Read the model definition and answer for the solid it produces. Units are mm, in the model's axes. Face numbers are marked on the shaded views. A direction names the side the tool comes from. Coordinates: 2 decimals unless noted, no trailing zeros. Write each loop counter-clockwise with the first axis right and the second up, starting at its lowest first coordinate (ties: lowest second). Pieces come first, ordered by that corner, then holes. Notation, with made-up numbers: (8, 8) -> (44, 8) arc R6 cw to (44, 15) -> close; hole circle Ø7 at (31.25, -17.5). An arc over 180 degrees is marked (long way). Return JSON: item names as keys, results as strings.
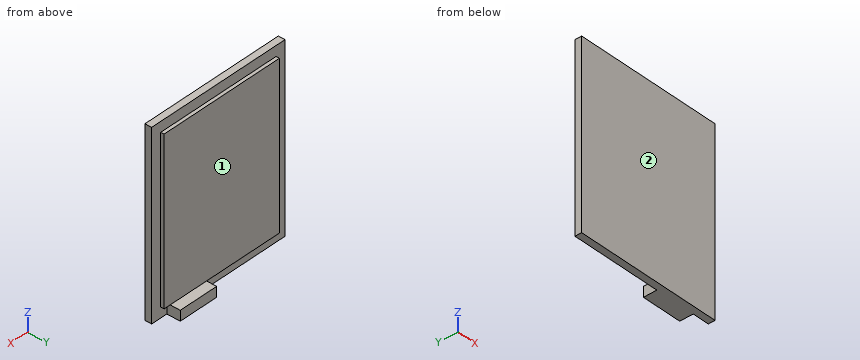
from build123d import *

# Parameters (mm, degrees)
SCHIZZO1_W                   = 44
SCHIZZO1_H                   = 54
ESTRUSIONE_ESTRUSIONE1_DEPTH = 2
SCHIZZO2_W                   = 38
SCHIZZO2_H                   = 48
ESTRUSIONE_ESTRUSIONE2_DEPTH = 1
SCHIZZO3_W                   = 12
SCHIZZO3_H                   = 3
ESTRUSIONE_ESTRUSIONE3_DEPTH = 4


with BuildPart() as part:
    # Schizzo1 → Estrusione-Estrusione1 (new body)
    with BuildSketch(Plane(origin=(0, 0, 0), x_dir=(1, 0, 0), z_dir=(0, 1, 0))):
        with Locations((9.928073705, -8.029830108)):
            Rectangle(SCHIZZO1_W, SCHIZZO1_H)
    extrude(amount=ESTRUSIONE_ESTRUSIONE1_DEPTH)

    # Schizzo2 → Estrusione-Estrusione2 (add)
    with BuildSketch(Plane(origin=(0, 2, 0), x_dir=(1, 0, 0), z_dir=(0, 1, 0))):
        with Locations((9.928073705, -8.029830108)):
            Rectangle(SCHIZZO2_W, SCHIZZO2_H)
    extrude(amount=ESTRUSIONE_ESTRUSIONE2_DEPTH)

    # Schizzo3 → Estrusione-Estrusione3 (add)
    with BuildSketch(Plane(origin=(0, 2, 0), x_dir=(1, 0, 0), z_dir=(0, 1, 0))):
        with Locations((20.928073705, 17.470169892)):
            Rectangle(SCHIZZO3_W, SCHIZZO3_H)
    extrude(amount=ESTRUSIONE_ESTRUSIONE3_DEPTH)


solid = part.part
1. The part is cut by section C-C (y = 4). Determine the outline of the cut face in (x, z).
Taken from the geometry:
{"outline": "(14.93, -18.97) -> (26.93, -18.97) -> (26.93, -15.97) -> (14.93, -15.97) -> close"}
2. Consider L1, parallel to Y at x = -4, z = -12; L2, parallel to Z at x = 19.5, y = 5.4; L3, parallel to Y at x = 29, z = 31.5. Determine where each line is inside the solid, lowest interval first.
Taken from the geometry:
{"L1": "y = 0 to 3", "L2": "z = -18.97 to -15.97", "L3": "y = 0 to 2"}
3. Flat-ended cylindrical pins translate along their axes: pin 1 Ø0.8 at (y, z) = (2.5, 6.5) entering from +X; pin 2 Ø0.8 at (x, y) = (28, 2.5) entering from -Z; pin 3 Ø2.5 at (y, z) = (3.5, -17.5) entering from +X. Find the tip coordinate at first contact, or state that the pin passes through.
Taken from the geometry:
{"pin 1": "stops at x = 28.93", "pin 2": "stops at z = -15.97", "pin 3": "stops at x = 26.93"}
4. The part is cut by section B-B (x = 20). Determine the outline of the cut face in (y, z).
Taken from the geometry:
{"outline": "(0, -18.97) -> (6, -18.97) -> (6, -15.97) -> (3, -15.97) -> (3, 32.03) -> (2, 32.03) -> (2, 35.03) -> (0, 35.03) -> close"}
5. A tool of negligible diameter and unlimited length cuts with its end or side. For the marked faces 1 and 2, from which of +Z, -Z, +X, -X, +Y, -Y can it reach the whole face along a straight path? Write none if from no direction.
Taken from the geometry:
{"face 1": "+Z, +X, -X, +Y", "face 2": "+Z, -Z, +X, -X, -Y"}
6. The part is cut by section A-A (z = -10.5). Determine the outline of the cut face in (x, y).
Taken from the geometry:
{"outline": "(-12.07, 0) -> (31.93, 0) -> (31.93, 2) -> (28.93, 2) -> (28.93, 3) -> (-9.07, 3) -> (-9.07, 2) -> (-12.07, 2) -> close"}
